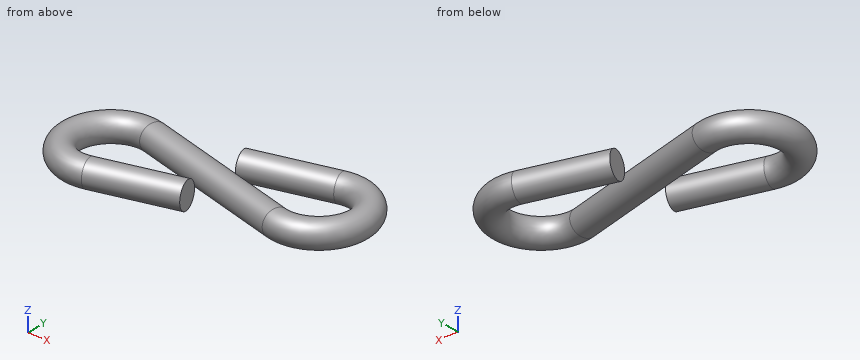
from build123d import *

# Parameters (mm, degrees)
SWEEP_1_PROFILE_R = 3


with BuildPart() as part:
    # По траектории1: sweep along a path in Эскиз1
    with BuildLine(Plane.XY) as sweep_1_path:
        Line((0, 7.5), (18.613206798, 12.48739373))
        ThreePointArc((18.613206798, 12.48739373), (30, 3.75), (18.613206798, -4.98739373))
        Line((18.613206798, -4.98739373), (0, 0))
        Line((0, 0), (-18.613206798, 4.98739373))
        ThreePointArc((-18.613206798, 4.98739373), (-30, -3.75), (-18.613206798, -12.48739373))
        Line((-18.613206798, -12.48739373), (0, -7.5))
    # По траектории1 profile (on start of the path) → По траектории1 (sweep)
    with BuildSketch(Plane(origin=(0, 7.5, 0), x_dir=(-0.25881904510251785, 0.9659258262890691, 0), z_dir=(0.9659258262890691, 0.25881904510251785, 0))):
        Circle(SWEEP_1_PROFILE_R)
    sweep(path=sweep_1_path.line)


solid = part.part
Model file for the job. Use its own axes, mm. Coordinates: 2 decimals unless noted, no trailing zeros. Loops run counter-clockwise (first coordinate to the right, second up) from the corner with the lowest first, then second, coordinate; pieces in that order, holes last. Notation, with made-up numbers: (49, -13) -> (102, -13) arc R26 ccw to (102, 20) -> close; hole circle Ø3 at (15, 7). An arc over 180 degrees is marked (long way). Use one line per item in the form item = value. Start each with the question number.
(1) Cut at A-A on z = -1.5. Give the cut face in (x, y).
(2) Cut at B-B on y = -6.5. Give the number of separate pieces and of enclosed holes in the cut face, and give its area (3 significant figures).
(3) Probe probe 1 along Y at (x, z) = (25.5, -1.25); probe 2 along Y at (x, z) = (10, -1.5); probe 3 along Y at (x, z) = (-29, 1.5). List the from-to ranges inside material, lowest first. Write a range as from..to.
(4) Cut at C-C on z = 1.25. Give the cut face in (x, y), and give its area (3 significant figures).
(5) Flat gauge pins, fed straight in: pin 1 (5 mm diameter, centred on x = 0.5, y = -0.5, fed in from -Z); pin 2 (8 mm diameter, centred on x = 13, y = 2, fed in from +Z); pin 3 (2 mm diameter, centred on y = 8.5, z = 1.5, fed in from +X); pin 4 (3 mm diameter, centred on y = -5, z = 1.5, fed in from -X). Where does each tip first touch, or does it go through?
Values:
q1.outline = (-19.29, -9.98) arc R6.45 cw (long way) to (-19.29, 2.48) -> (17.94, -7.5) arc R11.64 ccw (long way) to (17.94, 15) -> (-0.67, 10.01) -> (0.67, 4.99) -> (19.29, 9.98) arc R6.45 cw (long way) to (19.29, -2.48) -> (-17.94, 7.5) arc R11.64 ccw (long way) to (-17.94, -15) -> (0.67, -10.01) -> (-0.67, -4.99) -> close
q2.separate_pieces = 3
q2.enclosed_holes = 0
q2.area = 124 mm2
q3.probe_1 = -7.11..-0.64, 8.14..14.61
q3.probe_2 = -5.37..0.01, 7.49..12.87
q3.probe_3 = -12.17..4.67
q4.outline = (-19.32, -9.85) arc R6.32 cw (long way) to (-19.32, 2.35) -> (17.91, -7.62) arc R11.77 ccw (long way) to (17.91, 15.12) -> (-0.71, 10.13) -> (0.71, 4.87) -> (19.32, 9.85) arc R6.32 cw (long way) to (19.32, -2.35) -> (-17.91, 7.62) arc R11.77 ccw (long way) to (-17.91, -15.12) -> (0.71, -10.13) -> (-0.71, -4.87) -> close
q4.area = 782 mm2
q5.pin_1 = -3
q5.pin_2 = 2.71
q5.pin_3 = 32.19
q5.pin_4 = -32.98
